Work out the finished part from the listing and answer in its coordinate system (mm). Face numbers are marked on the shaded views. A direction names the side the tool comes from. Give positions to 0.01 mm unless a question says otherwise; leave off trailing zeros. Loops run counter-clockwise (first coordinate to the right, second up) from the corner with the lowest first, then second, coordinate; pieces in that order, holes last. Notation, with made-up numbers: (10.5, 49) - (56.5, 49) arc R22 cw to (56.5, 86) - close; hole circle Ø10 at (83, -38). An arc over 180 degrees is marked (long way). One line per item, written item: value.
from build123d import *

# Parameters (mm, degrees)
F1_DEPTH       = 6.35
F2_R           = 3.81
F3_DEPTH       = 6.35
F5_D           = 2.032
F5_CSINK_D     = 3.175
F5_CSINK_ANGLE = 82
F7_D           = 2.032


with BuildPart() as f1:
    # F0 (on Front) → F1 (new body)
    with BuildSketch(Plane.XZ):
        with BuildLine():
            Line((3.550874937, 5.2643885857), (0, 0))
            Line((0, 0), (0, -6.35))
            ThreePointArc((0, -6.35), (2.9811444237, -5.6067172147), (5.2643885857, -3.550874937))
            Line((5.2643885857, -3.550874937), (6.35, -1.9413898273))
            Line((6.35, -1.9413898273), (6.35, 0))
            ThreePointArc((6.35, 0), (5.6067172147, 2.9811444237), (3.550874937, 5.2643885857))
        make_face()
        with BuildLine():
            Line((0, -6.35), (0, 0))
            Line((0, 0), (3.550874937, 5.2643885857))
            ThreePointArc((3.550874937, 5.2643885857), (-1.2116371206, 6.2333326149), (-5.2643885857, 3.550874937))
            ThreePointArc((-5.2643885857, 3.550874937), (-6.0725352004, 1.856560325), (-6.35, 0))
            ThreePointArc((-6.35, 0), (-4.4901280605, -4.4901280605), (0, -6.35))
        make_face()
        with BuildLine():
            ThreePointArc((5.2643885857, -3.550874937), (2.9811444237, -5.6067172147), (0, -6.35))
            Line((0, -6.35), (0, -15.24))
            ThreePointArc((0, -15.24), (4.4901280605, -17.0998719395), (6.35, -21.59))
            Line((6.35, -21.59), (6.35, -1.9413898273))
            Line((6.35, -1.9413898273), (5.2643885857, -3.550874937))
        make_face()
        with BuildLine():
            Line((0, -15.24), (0, -6.35))
            ThreePointArc((0, -6.35), (-4.4901280605, -4.4901280605), (-6.35, 0))
            Line((-6.35, 0), (-6.35, -21.59))
            ThreePointArc((-6.35, -21.59), (-4.4901280605, -17.0998719395), (0, -15.24))
        make_face()
        with BuildLine():
            ThreePointArc((-5.2643885857, 3.550874937), (-1.2116371206, 6.2333326149), (3.550874937, 5.2643885857))
            ThreePointArc((3.550874937, 5.2643885857), (5.6067172147, 2.9811444237), (6.35, 0))
            Line((6.35, 0), (6.35, -1.9413898273))
            Line((6.35, -1.9413898273), (27.9899881828, 30.1412120116))
            ThreePointArc((27.9899881828, 30.1412120116), (26.2764745341, 38.9564755344), (17.4612110113, 37.2429618857))
            Line((17.4612110113, 37.2429618857), (-5.2643885857, 3.550874937))
        make_face()
        with BuildLine():
            ThreePointArc((6.35, -21.59), (4.4901280605, -17.0998719395), (0, -15.24))
            Line((0, -15.24), (0, -21.59))
            Line((0, -21.59), (0, -27.94))
            ThreePointArc((0, -27.94), (4.4901280605, -26.0801280605), (6.35, -21.59))
        make_face()
        with BuildLine():
            Line((0, -21.59), (0, -15.24))
            ThreePointArc((0, -15.24), (-4.4901280605, -17.0998719395), (-6.35, -21.59))
            ThreePointArc((-6.35, -21.59), (-4.4901280605, -26.0801280605), (0, -27.94))
            Line((0, -27.94), (0, -21.59))
        make_face()
        with BuildLine():
            ThreePointArc((0, -27.94), (-4.4901280605, -26.0801280605), (-6.35, -21.59))
            Line((-6.35, -21.59), (-6.35, -34.29))
            ThreePointArc((-6.35, -34.29), (0, -40.64), (6.35, -34.29))
            Line((6.35, -34.29), (6.35, -21.59))
            ThreePointArc((6.35, -21.59), (4.4901280605, -26.0801280605), (0, -27.94))
        make_face()
    extrude(amount=F1_DEPTH)

    # F2 (on face) → F3 (join)
    with BuildSketch(Plane.XZ.offset(6.35)):
        with Locations((0, -21.59)):
            Circle(F2_R)
    extrude(amount=F3_DEPTH)

    # F5 (through all)
    with Locations(Plane.XZ.offset(12.7)):
        with Locations((0, -21.59)):
            CounterSinkHole(F5_D / 2, F5_CSINK_D / 2, counter_sink_angle=F5_CSINK_ANGLE)

    # F7 (through all)
    with Locations(Plane.XZ.offset(6.35)):
        with Locations((0, -34.29)):
            Hole(F7_D / 2)


solid = f1.part
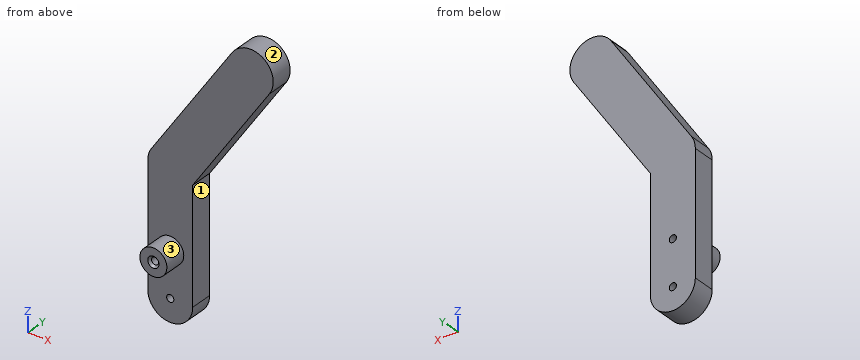
1. Section B-B (y = -3.5) is taken. Write down the section's boundary in (x, z), and give its area (3 significant figures).
Output:
outline: (-6.35, -34.29) arc R6.35 ccw to (6.35, -34.29) - (6.35, -1.94) - (27.99, 30.14) arc R6.35 ccw to (17.46, 37.24) - (-5.26, 3.55) arc R6.35 ccw to (-6.35, 0) - close; hole circle Ø2.03 at (0, -34.29); hole circle Ø2.03 at (0, -21.59)
area: 1,070 mm²
2. Find the intervals of material crossed by line 1 along Z through (x, y) = (0, -9.5); line 2 along Z through (x, y) = (0.5, -5); line 3 along Z through (x, y) = (0, -5.75), in increasing order.
Output:
line 1: z = -25.4 to -22.61, -20.57 to -17.78
line 2: z = -40.62 to -35.17, -33.41 to -22.47, -20.71 to 12.1
line 3: z = -40.64 to -35.31, -33.27 to -22.61, -20.57 to 11.36
3. Section D-D (z = -3) is taken. Write down the section's boundary in (x, y).
Output:
outline: (-6.35, -6.35) - (6.35, -6.35) - (6.35, 0) - (-6.35, 0) - close
4. For the marked faces 1, 2 and 3, determine the directions among +Z, -Z, +X, -X, +Y, -Y from which every point of the face is accessible in a straight line to the end or side of a thin tool.
Output:
face 1: -Z, +X, +Y, -Y
face 2: +Y, -Y
face 3: -Y
5. Section C-C (x = 0) is taken. Write down the section's boundary in (y, z), and give its area (3 significant figures).
Output:
outline: (-12.7, -25.4) - (-6.35, -25.4) - (-6.35, -33.27) - (0, -33.27) - (0, -22.61) - (-12.04, -22.61) - (-12.7, -23.18) - close; (-12.7, -20) - (-12.04, -20.57) - (0, -20.57) - (0, 11.36) - (-6.35, 11.36) - (-6.35, -17.78) - (-12.7, -17.78) - close; (-6.35, -40.64) - (0, -40.64) - (0, -35.31) - (-6.35, -35.31) - close
area: 339 mm²
6. Flat-ended cylindrical pins translate along their axes: pin 1 Ø10 at (x, z) = (2.5, 10) entering from -Y; pin 2 Ø6 at (y, z) = (-1.5, -26.5) entering from +X; pin 3 Ø3 at (y, z) = (-4, 10) entering from +X. Find the tip coordinate at first contact, or state that the pin passes through.
Output:
pin 1: stops at y = -6.35
pin 2: stops at x = 6.35
pin 3: stops at x = 15.42
7. Section A-A (z = -21.59) is taken. Write down the section's boundary in (x, y), and give its area (3 significant figures).
Output:
outline: (-6.35, -6.35) - (-3.81, -6.35) - (-3.81, -12.7) - (-1.59, -12.7) - (-1.02, -12.04) - (-1.02, 0) - (-6.35, 0) - close; (1.02, -12.04) - (1.59, -12.7) - (3.81, -12.7) - (3.81, -6.35) - (6.35, -6.35) - (6.35, 0) - (1.02, 0) - close
area: 103 mm²
